Geometry check sheet. Reference: the model listing, model coordinates, mm. A direction names the side the tool comes from. Round coordinates to 2 decimals unless told otherwise and drop trailing zeros. Order: outer loops, then holes, each group sorted by start corner. A loop starts at its lowest first (then second) coordinate and runs counter-clockwise, first axis right, second up. Notation, with made-up numbers: (-34, 34) -> (11, 34) arc R28 ccw to (11, 56) -> close; hole circle Ø7 at (24.5, 1). An arc over 180 degrees is marked (long way). Answer as a JSON object with one key per item and string values. Group by question number.
from build123d import *

# Parameters (mm, degrees)
F1_DEPTH = 4
F3_DEPTH = 4.0010001


with BuildPart() as f1:
    # F0 (on Front) → F1 (new body)
    with BuildSketch(Plane.XZ):
        with BuildLine():
            Line((-2.25, 21.0164487362), (-2.25, 0))
            Line((-2.25, 0), (2.25, 0))
            Line((2.25, 0), (2.25, 21.0164487362))
            add(Edge.make_bspline(
                [(0, 29.0521112765), (0.3695458095, 28.9210731345), (1.3268018727, 28.5816373926), (1.8741963924, 25.3153750937), (2.1164189838, 22.5445206862), (2.25, 21.0164487362)],
                knots=[0, 0, 0, 0, 0.219983541, 0.5698361963, 1, 1, 1, 1], degree=3))
            add(Edge.make_bspline(
                [(0, 29.0521112765), (-0.3695458095, 28.9210731345), (-1.3268018727, 28.5816373926), (-1.8741963924, 25.3153750937), (-2.1164189838, 22.5445206862), (-2.25, 21.0164487362)],
                knots=[0, 0, 0, 0, 0.219983541, 0.5698361963, 1, 1, 1, 1], degree=3))
        make_face()
        with BuildLine():
            Line((-1, 13), (-1, 22))
            ThreePointArc((-1, 22), (0, 23), (1, 22))
            Line((1, 22), (1, 13))
            ThreePointArc((1, 13), (0, 12), (-1, 13))
        make_face(mode=Mode.SUBTRACT)
        Polygon((-2.25, 0), (-4.5, 0), (-4.5, -50), (4.5, -50), (4.5, 0), (2.25, 0), align=None)
    extrude(amount=F1_DEPTH)

    # F2 (on face) → F3 (cut, through all)
    with BuildSketch(Plane.XZ.offset(4)):
        with BuildLine():
            Line((4.5, 0), (2.25, 0))
            ThreePointArc((2.25, 0), (2.9090097423, -1.5909902577), (4.5, -2.25))
            Line((4.5, -2.25), (4.5, 0))
        make_face()
        with BuildLine():
            Line((-4.5, 0), (-4.5, -2.25))
            ThreePointArc((-4.5, -2.25), (-2.9090097423, -1.5909902577), (-2.25, 0))
            Line((-2.25, 0), (-4.5, 0))
        make_face()
    extrude(amount=-F3_DEPTH, mode=Mode.SUBTRACT)


solid = f1.part
Item 1: Sectioned sample at A-A, the plane z = 6.5. Enter the section's corners in (x, y).
Item 2: Set-up check for faces 1 (the cylindrical face through (0, -2, 12)), 2 (the flat face through (2.25, -2, 10)), 3 (the flat face through (0, -4, -19)): record each of +Z, -Z, +X, -X, +Y, -Y from which the full face is reachable in a straight line by a thin tool's end or side.
Item 3: Depth check by flat-ended pin: pin 1 Ø1.5 at (x, z) = (-0.5, 15) entering from -Y. Enter the tip coordinate at first touch or a pass-through.
Item 4: Thickness scan on L1, parallel to Z at x = 0, y = -1.65; L2, parallel to X at y = -1, z = 20; L3, parallel to Z at x = 0.75, y = -1.45. Record the ranges inside material, lowest first.
Item 5: Mould release check, pull along X, two halves, no side actions. Record for faces 4 (the cylindrical face through (0, -2, 23)), 5 (the flat face through (-1, -2, 17)), 6 (the flat face through (-2.25, -2, 11)), 7 (the flat face through (0, -2, -50)): pulls with the +X half, pulls with the -X half, needs draft (parallel to the pull), parting line crosses it, or undercut.
Result:
{
 "1": {"outline": "(-2.25, -4) -> (2.25, -4) -> (2.25, 0) -> (-2.25, 0) -> close"},
 "2": {"face 1": "+Y, -Y", "face 2": "+Z, +X, +Y, -Y", "face 3": "+Z, -Z, +X, -X, -Y"},
 "3": {"pin 1": "stops at y = -4"},
 "4": {"L1": "z = -50 to 12, 23 to 29.05", "L2": "x = -2.25 to -1, 1 to 2.25", "L3": "z = -50 to 12.34, 22.66 to 28.69"},
 "5": {"face 4": "undercut", "face 5": "undercut", "face 6": "pulls with the -X half", "face 7": "needs draft"}
}
